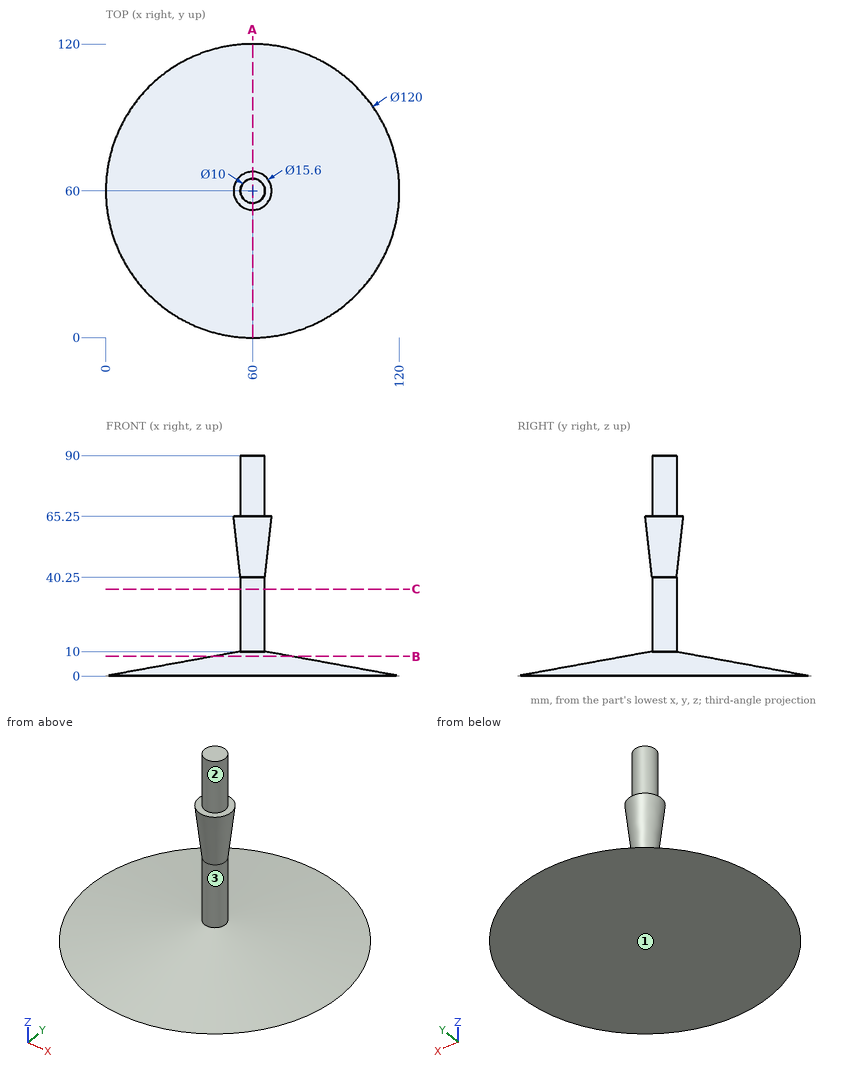
The figure shows three views and two pictorial views of one solid part (mm, origin at its lowest corner). Answer the questions. Round coordinates to 2 decimals unless told otherwise and drop trailing zeros. Write each loop counter-clockwise with the first axis right and the second up, starting at its lowest first coordinate (ties: lowest second). Pieces come first, ordered by that corner, then holes. Notation, with made-up numbers: (-10, 41.5) - (46, 41.5) arc R19 ccw to (46, 47.5) - close; hole circle Ø9 at (61.5, 51). An arc over 180 degrees is marked (long way). Answer in a Markdown table with one row per item. Add a question column.
1. Find the intervals of material crossed by line 1 along Y through (x, z) = (58, 44); line 2 along Z through (x, y) = (39, 69); line 3 along X through (y, z) = (63, 85), in increasing order. Write a range as from..to.
2. A cutting plane is placed at A-A, the plane x = 60. Determine the outline of the cut face in (y, z).
3. The mould has two halves that part along Z. Classify the marked faces 1, 2 and 3: +Z half, -Z half, draft (parallel to the pull), parting line (faces both ways), or undercut.
4. A cutting plane is placed at C-C, the plane z = 35.5. Determine the outline of the cut face in (x, y), and give its area (3 significant figures).
5. Given pin 1 (6 mm diameter, centred on x = 39, y = 63.5, fed in from +Z); pin 2 (5 mm diameter, centred on x = 25, y = 91.5, fed in from +Z); pin 3 (2 mm diameter, centred on x = 41.5, y = 33.5, fed in from +Z); pin 4 (4 mm diameter, centred on x = 51, z = 42.5, fed in from +Y), each flat-ended and moving along its own axis, determine where each tip first touches the part or whether it passes through.
6. A cutting plane is placed at B-B, the plane z = 8. Determine the outline of the cut face in (x, y).
Worked out:
| question | item | result |
|---|---|---|
| 1 | line 1 | 54.96..65.04 |
| 1 | line 2 | 0..6.76 |
| 1 | line 3 | 56..64 |
| 2 | outline | (0, 0) - (120, 0) - (65, 10) - (65, 40.25) - (67.8, 65.25) - (65, 65.25) - (65, 90) - (55, 90) - (55, 65.25) - (52.2, 65.25) - (55, 40.25) - (55, 10) - close |
| 3 | face 1 | -Z half |
| 3 | face 2 | draft |
| 3 | face 3 | undercut |
| 4 | outline | circle Ø10 at (60, 60) |
| 4 | area | 78.5 mm^2 |
| 5 | pin 1 | z = 7.58 |
| 5 | pin 2 | z = 2.8 |
| 5 | pin 3 | z = 5.21 |
| 5 | pin 4 | through |
| 6 | outline | circle Ø32 at (60, 60) |
